Here's the drawing with two shaded views (mm, measured from the low corner). I have some questions. A direction names the side the tool comes from. Coordinates: 2 decimals unless noted, no trailing zeros. Order: outer loops, then holes, each group sorted by start corner. A loop starts at its lowest first (then second) coordinate and runs counter-clockwise, first axis right, second up. Notation, with made-up numbers: (45.5, 50) - (77.5, 50) arc R9 cw to (77.5, 59) - close; hole circle Ø9 at (-28.5, -14.75). An arc over 180 degrees is marked (long way). Answer as a JSON object with one key per item and string values. Group by question number.
(1) Will these pins go through, and if not, where does the flat tip stop? P1, Ø1.2, axis at x = 3.5, y = 7, coming from the +Z side; P2, Ø1.9, axis at y = 8, z = 9.5, coming from the +X side; P3, Ø2, axis at x = 8.5, y = 1, coming from the +Z side.
(2) Imagine slicing it at A-A, the plane z = 12.75. Write out the boundary of the cut face in (x, y) (1 decimal).
(3) Imagine slicing it at D-D, the plane z = 2.75. Write out the boundary of the cut face in (x, y).
(4) Imagine slicing it at B-B, the plane x = 11.5. Write out the boundary of the cut face in (y, z) (1 decimal).
(5) Imagine slicing it at C-C, the plane y = 7. Write out the boundary of the cut face in (x, z) (3 decimals).
(6) Please list where these lines run through material, in increasing order: probe 1 along X at (y, z) = (10, 9.5) (1 decimal); probe 2 along Y at (x, z) = (15.25, 16.5); probe 3 along Z at (x, y) = (7.25, 9.25).
(7) Which directions (+Z, -Z, +X, -X, +Y, -Y) give clear straight access to the entire face, cutting with the end or side of a thin tool? Please do the marked faces 4 and 5.
(8) We'd pull the mould along X, two halves only. Please class the marked faces 1, 2 and 3: pulls with the +X half, pulls with the -X half, needs draft (parallel to the pull), parting line crosses it, or undercut.
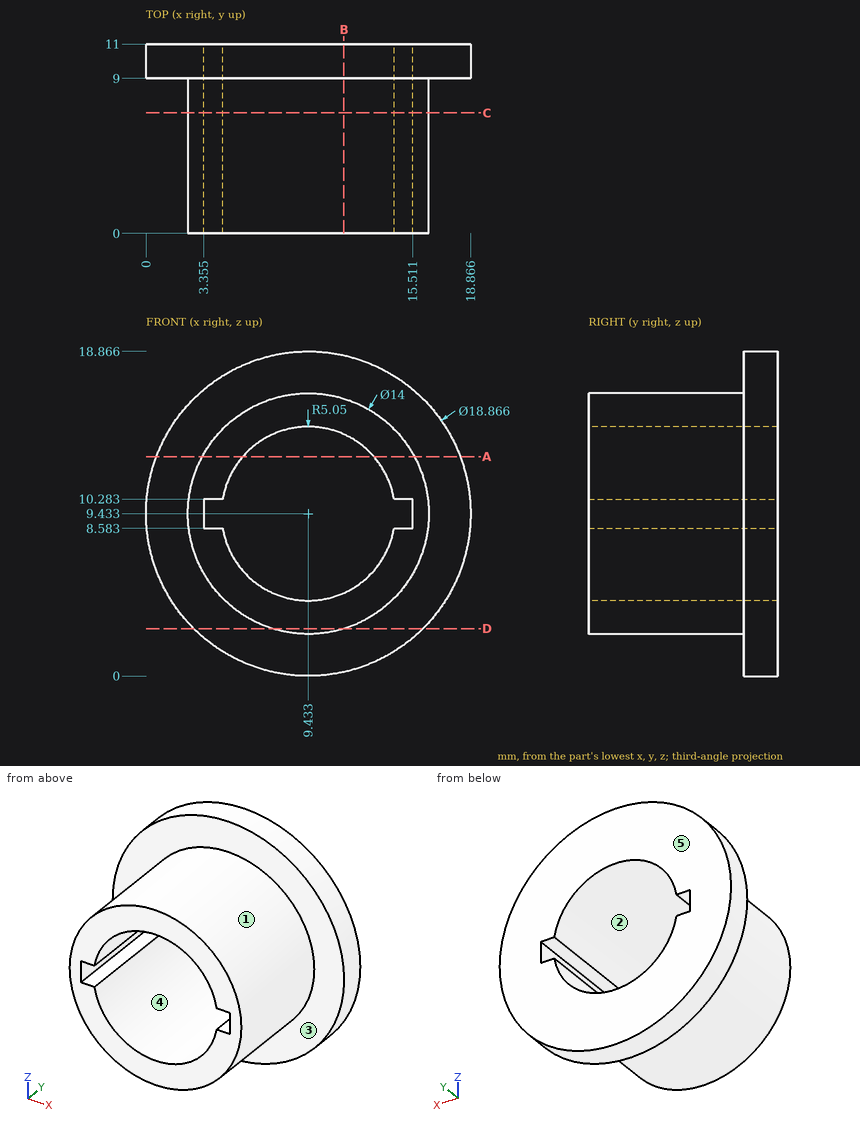
Result set:
{
 "1": {"P1": "stops at z = 13.97", "P2": "stops at x = 16.43", "P3": "stops at z = 16.43"},
 "2": {"outline": "(0.6, 9) - (3.3, 9) - (3.3, 0) - (5.6, 0) - (5.6, 11) - (0.6, 11) - close; (13.2, 0) - (15.6, 0) - (15.6, 9) - (18.3, 9) - (18.3, 11) - (13.2, 11) - close"},
 "3": {"outline": "(2.78, 9) - (7.35, 9) - (7.35, 0) - (11.52, 0) - (11.52, 9) - (16.09, 9) - (16.09, 11) - (2.78, 11) - close"},
 "4": {"outline": "(0, 2.7) - (9, 2.7) - (9, 0.2) - (11, 0.2) - (11, 4.8) - (0, 4.8) - close; (0, 14) - (11, 14) - (11, 18.6) - (9, 18.6) - (9, 16.1) - (0, 16.1) - close"},
 "5": {"outline": "circle Ø14 at (9.433, 9.433); hole (3.355, 8.583) - (4.455, 8.583) arc R5.05 ccw to (14.411, 8.583) - (15.511, 8.583) - (15.511, 10.283) - (14.411, 10.283) arc R5.05 ccw to (4.455, 10.283) - (3.355, 10.283) - close"},
 "6": {"probe 1": "x = 0 to 3.4, 15.5 to 18.9", "probe 2": "y = 9 to 11", "probe 3": "z = 0.26 to 4.88, 13.99 to 18.61"},
 "7": {"face 4": "+Y, -Y", "face 5": "+Z, -Z, +X, -X, +Y"},
 "8": {"face 1": "parting line crosses it", "face 2": "undercut", "face 3": "needs draft"}
}
